For this review, use the dimensioned drawing (mm, ordinates from the lowest corner) and the shaded views. Coordinates: 2 decimals unless noted, no trailing zeros. Loops run counter-clockwise (first coordinate to the right, second up) from the corner with the lowest first, then second, coordinate; pieces in that order, holes last. Notation, with made-up numbers: (52.5, -32) - (58.5, -32) arc R15 cw to (58.5, -13) - close; hole circle Ø10 at (38.25, 88.5). An arc over 180 degrees is marked (long way). One line per item, written item: value. Start each with the question number.
1. We need section A-A, the plane y = 3. Give the boundary of the cut face in (x, z), then the cut area to 3 significant figures.
2. We need section D-D, the plane z = 8. Give the boundary of the cut face in (x, y).
3. Insertion check: P1, Ø1.5, axis at x = 3, y = 3, coming from the +Z side. The pin has a flat end and moves straight along its axis. Give the tip position at first contact, or say it passes through.
4. We need section C-C, the plane z = 42. Give the boundary of the cut face in (x, y).
5. To check wall thickness, follow line 1 (Y direction, x = 3, z = 4.2); line 2 (X direction, y = 3.1, z = 16); line 3 (Z direction, x = 3, y = 4.45). State the ranges of each line that lie inside material, in increasing order.
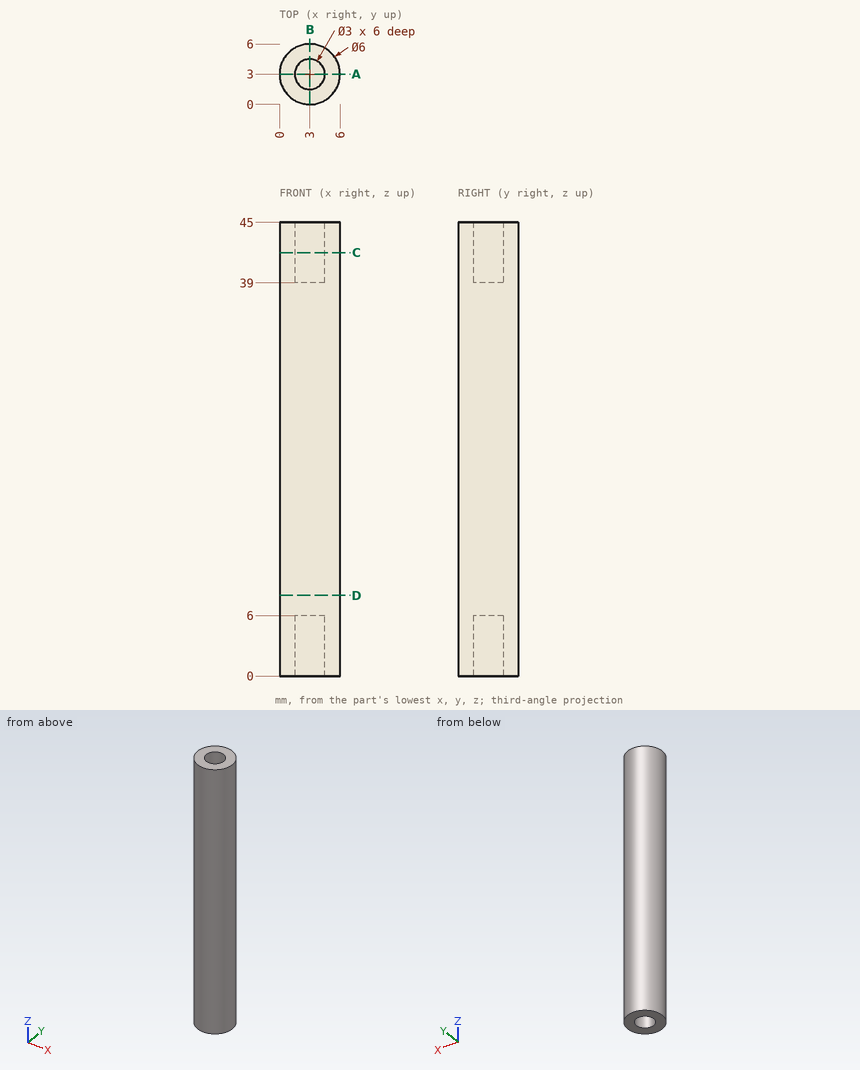
Findings below:
1. outline: (0, 0) - (1.5, 0) - (1.5, 6) - (4.5, 6) - (4.5, 0) - (6, 0) - (6, 45) - (4.5, 45) - (4.5, 39) - (1.5, 39) - (1.5, 45) - (0, 45) - close
1. area: 234 mm2
2. outline: circle Ø6 at (3, 3)
3. P1: z = 39
4. outline: circle Ø6 at (3, 3); hole circle Ø3 at (3, 3)
5. line 1: 0 to 1.5, 4.5 to 6
5. line 2: 0 to 6
5. line 3: 6 to 39
